```python
from build123d import *

# Parameters (mm, degrees)
SKETCH_1_W         = 42
SKETCH_1_H         = 38
TOP_DEPTH          = 1
DHT22_WINDOW_REACH = 30.337
SKETCH_2_W         = 20.5
SKETCH_2_H         = 15.5


with BuildPart() as part:
    # 스케치1 → Top (new body)
    with BuildSketch(Plane(origin=(0, 0, 0), x_dir=(1, 0, 0), z_dir=(0, 1, 0))):
        Rectangle(SKETCH_1_W, SKETCH_1_H)
    extrude(amount=TOP_DEPTH)

    # 스케치2 → DHT22_window (cut, up to next)
    with BuildSketch(Plane(origin=(0, 1, 0), x_dir=(1, 0, 0), z_dir=(0, 1, 0)), mode=Mode.PRIVATE) as dht22_window_sk1:
        with Locations((2, -2)):
            Rectangle(SKETCH_2_W, SKETCH_2_H)
    dht22_window_tool1 = extrude(dht22_window_sk1.sketch, amount=-DHT22_WINDOW_REACH, mode=Mode.PRIVATE) & part.part
    add(dht22_window_tool1.solids().sort_by_distance((2, 1, 2))[0], mode=Mode.SUBTRACT)


solid = part.part
```
Check sheet for the modelled part. Datum: model origin and axes. Units: mm. A direction names the side the tool comes from. Give positions to 0.01 mm unless a question says otherwise; leave off trailing zeros. Write each loop counter-clockwise with the first axis right and the second up, starting at its lowest first coordinate (ties: lowest second). Pieces come first, ordered by that corner, then holes. Notation, with made-up numbers: (85, -1.75) - (92, -1.75) arc R26 ccw to (92, 29.25) - close; hole circle Ø5 at (29, 3.25). An arc over 180 degrees is marked (long way). Answer as a JSON object with one key per item and string values. Group by question number.
1) Access from +Z, -Z, +X, -X, +Y, -Y to the whole of each face (thin tool, end or side, straight path). Record for faces 5 (the face through (-0.3, 0.5, 19)), 6 (the face through (1.9, 0.5, -5.75)).
2) Depth check by flat-ended pin: P1, Ø2, axis at x = 14, z = -2.5, coming from the -Y side. Enter the tip coordinate at first touch or a pass-through.
3) Sectioned sample at C-C (y = 0.85). Record the cut outline in (x, z), then the cut area to 3 significant figures.
4) Sectioned sample at B-B (z = -5). Record the cut outline in (x, y).
5) Sectioned sample at A-A (x = 3.5). Record the cut outline in (y, z).
6) Thickness scan on probe 1 along Z at (x, y) = (7, 0.4); probe 2 along X at (y, z) = (0.2, 3). Record the ranges inside material, lowest first. Write a range as from..to.
7) Release check for a two-part mould opening along X. For faces 1 (the face through (21, 0.5, 0.3)), 2 (the face through (0, 1, -9)), 3 (the face through (1.9, 0.5, 9.75)), 4 (the face through (12.25, 0.5, 2.1)) record: pulls with the +X half, pulls with the -X half, needs draft (parallel to the pull), parting line crosses it, or undercut.
Geometry results:
{
 "1": {"face 5": "+Z, +X, -X, +Y, -Y", "face 6": "+Y, -Y"},
 "2": {"P1": "stops at y = 0"},
 "3": {"outline": "(-21, -19) - (21, -19) - (21, 19) - (-21, 19) - close; hole (-8.25, -5.75) - (12.25, -5.75) - (12.25, 9.75) - (-8.25, 9.75) - close", "area": "1,280 mm^2"},
 "4": {"outline": "(-21, 0) - (-8.25, 0) - (-8.25, 1) - (-21, 1) - close; (12.25, 0) - (21, 0) - (21, 1) - (12.25, 1) - close"},
 "5": {"outline": "(0, -19) - (1, -19) - (1, -5.75) - (0, -5.75) - close; (0, 9.75) - (1, 9.75) - (1, 19) - (0, 19) - close"},
 "6": {"probe 1": "z = -19..-5.75, 9.75..19", "probe 2": "x = -21..-8.25, 12.25..21"},
 "7": {"face 1": "pulls with the +X half", "face 2": "needs draft", "face 3": "undercut", "face 4": "undercut"}
}
